from build123d import *

# Parameters (mm, degrees)
SKETCH_2_R              = 31
EXTRUDE_1_DEPTH         = 170
HOLE_WIZARD_M24_1_D     = 21
HOLE_WIZARD_M24_1_DEPTH = 40
HOLE_WIZARD_M24_1_TIP   = 6.3090365
CUT_EXTRUDE_START       = -40
SKETCH_6_R              = 15
CUT_EXTRUDE_1_DEPTH     = 54
CUT_EXTRUDE_START_2     = -25
CUT_EXTRUDE_2_DEPTH     = 151.561954876


with BuildPart() as part:
    # 草图2 → 凸台-拉伸1 (new body)
    with BuildSketch(Plane(origin=(0, 0, 0), x_dir=(0, 0, -1), z_dir=(1, 0, 0))):
        Circle(SKETCH_2_R)
    extrude(amount=EXTRUDE_1_DEPTH)

    # M24 螺纹孔1
    with Locations(Plane(origin=(170, 0, 0), x_dir=(0, 0, -1), z_dir=(1, 0, 0))):
        with Locations((0, 0)):
            Hole(HOLE_WIZARD_M24_1_D / 2, depth=HOLE_WIZARD_M24_1_DEPTH)
            with Locations((0, 0, -(HOLE_WIZARD_M24_1_DEPTH + HOLE_WIZARD_M24_1_TIP / 2))):  # 118° drill point
                Cone(0, HOLE_WIZARD_M24_1_D / 2, HOLE_WIZARD_M24_1_TIP, mode=Mode.SUBTRACT)

    # 草图6 → 切除-拉伸1 (cut)
    with BuildSketch(Plane(origin=(170, 0, 0), x_dir=(0, 0, -1), z_dir=(1, 0, 0)).offset(CUT_EXTRUDE_START)):
        Circle(SKETCH_6_R)
    extrude(amount=-CUT_EXTRUDE_1_DEPTH, mode=Mode.SUBTRACT)

    # 草图7 → 切除-旋转1 (revolve, cut)
    with BuildSketch(Plane.XY, mode=Mode.PRIVATE) as cut_revolve_1_sk:
        Polygon((0, 0), (76, 0), (76, 10), (0, 13.8), align=None)
    revolve(cut_revolve_1_sk.sketch.rotate(Axis((76, 0, 0), (1, 0, 0)), 270), axis=Axis((76, 0, 0), (1, 0, 0)), mode=Mode.SUBTRACT)

    # 草图8 → 切除-拉伸2 (cut, through all)
    with BuildSketch(Plane(origin=(0, 0, 0), x_dir=(1, 0, 0), z_dir=(0, 1, 0)).offset(CUT_EXTRUDE_START_2)):
        with BuildLine():
            Line((25, 5), (83, 5))
            ThreePointArc((83, 5), (88, 0), (83, -5))
            Line((83, -5), (25, -5))
            ThreePointArc((25, -5), (20, 0), (25, 5))
        make_face()
    extrude(amount=-CUT_EXTRUDE_2_DEPTH, mode=Mode.SUBTRACT)


solid = part.part
Source: CAD feature listing. Evaluate the final solid. Frame: model axes, mm. A direction names the side the tool comes from. Round coordinates to 2 decimals unless told otherwise and drop trailing zeros. Loops run counter-clockwise (first coordinate to the right, second up) from the corner with the lowest first, then second, coordinate; pieces in that order, holes last. Notation, with made-up numbers: (-31.5, 46.25) -> (-21.5, 46.25) arc R22 ccw to (-21.5, 73.25) -> close; hole circle Ø9 at (-4, 75.25). An arc over 180 degrees is marked (long way). Answer as a JSON object with one key per item and string values. Group by question number.
Q1. Section query C-C (x = 78.5). Output: boundary loops of the cut face in (y, z).
Q2. Access query for faces 1 (the flat face through (54, -25, 0)), 2 (the cylindrical face through (83.81, 30.736, 4.036)), 3 (the flat face through (76, -10, -3)). Directions: +Z, -Z, +X, -X, +Y, -Y. A direction counts if a zero-diameter tool reaches every point of the face in a straight line with its end or side. Return the directions, or none.
Q3. Section query D-D (x = 107). Output: boundary loops of the cut face in (y, z).
Q4. Section query B-B (z = 0). Output: boundary loops of the cut face in (x, y), plus the area to 3 significant figures.
Q5. Section query A-A (y = 0). Output: boundary loops of the cut face in (x, z), plus the area to 3 significant figures.
Q6. Mould query, pull axis X, two halves, no side actions, for faces 4 (the cylindrical face through (149.7, 3.2, 10)), 5 (the flat face through (170, -13, 0)), 6 (the cylindrical face through (88, -28, 0)), 7 (the conical face through (37.468, 3.582, -11.376)). Classes: pulls with the +X half, pulls with the -X half, needs draft (parallel to the pull), parting line crosses it, or undercut.
Q7. Ray query, line 1 (Y direction, x = 140, z = 0); line 2 (X direction, y = 14.5, z = -2.5); line 3 (Y direction, x = 114, z = 0). Return the intervals inside material, ascending. Write a range as from..to.
Q8. Contact query for flat-ended pins moving along their axis: P1, Ø12, axis at x = 72, y = -7, coming from the +Z side; P2, Ø3, axis at x = 136, y = -17.5, coming from the +Z side; P3, Ø1.7, axis at x = 55.5, y = -28, coming from the +Z side; P4, Ø2, axis at y = 20, z = 23, coming from the -X side. Output: stop coordinate, or through.
Completed:
{
 "1": {"outline": "(-30.59, -5) arc R31 ccw (long way) to (-30.59, 5) -> (-25, 5) -> (-25, -5) -> close; hole circle Ø30 at (0, 0)"},
 "2": {"face 1": "-Y", "face 2": "+X, -X", "face 3": "none"},
 "3": {"outline": "circle Ø62 at (0, 0); hole circle Ø30 at (0, 0)"},
 "4": {"outline": "(0, -31) -> (20, -31) -> (20, -25) -> (88, -25) -> (88, -31) -> (170, -31) -> (170, -10.5) -> (130, -10.5) -> (130, -15) -> (76, -15) -> (76, -10) -> (0, -13.8) -> close; (0, 13.8) -> (76, 10) -> (76, 15) -> (130, 15) -> (130, 10.5) -> (170, 10.5) -> (170, 31) -> (0, 31) -> close", "area": "5,860 mm²"},
 "5": {"outline": "(0, -31) -> (170, -31) -> (170, -10.5) -> (130, -10.5) -> (130, -15) -> (76, -15) -> (76, -10) -> (0, -13.8) -> close; (0, 13.8) -> (76, 10) -> (76, 15) -> (130, 15) -> (130, 10.5) -> (170, 10.5) -> (170, 31) -> (0, 31) -> close", "area": "6,270 mm²"},
 "6": {"face 4": "needs draft", "face 5": "pulls with the +X half", "face 6": "undercut", "face 7": "pulls with the -X half"},
 "7": {"line 1": "-31..-10.5, 10.5..31", "line 2": "0..76, 130..170", "line 3": "-31..-15, 15..31"},
 "8": {"P1": "z = 30.98", "P2": "z = 26.55", "P3": "z = 14.96", "P4": "x = 0"}
}
